Read the model definition and answer for the solid it produces. Units are mm, in the model's axes. A direction names the side the tool comes from. Coordinates: 2 decimals unless noted, no trailing zeros. Loops run counter-clockwise (first coordinate to the right, second up) from the corner with the lowest first, then second, coordinate; pieces in that order, holes last. Notation, with made-up numbers: (-4.75, 25.5) -> (15.25, 25.5) arc R3 ccw to (15.25, 30.5) -> close; hole circle Ø3 at (56, -34). An arc over 180 degrees is marked (long way). Answer in a Markdown table with one row per item.
```python
from build123d import *

# Parameters (mm, degrees)
SKETCH_1_R          = 10
SKETCH_1_R_2        = 1.65
EXTRUDE_1_DEPTH     = 3
SKETCH_2_R          = 3
EXTRUDE_2_DEPTH     = 80
CUT_EXTRUDE_1_DEPTH = 20


with BuildPart() as part:
    # 草图1 → 凸台-拉伸1 (new body)
    with BuildSketch(Plane.XY):
        Circle(SKETCH_1_R)
        with Locations((0, 7)):
            Circle(SKETCH_1_R_2, mode=Mode.SUBTRACT)
        with Locations((7, 0)):
            Circle(SKETCH_1_R_2, mode=Mode.SUBTRACT)
        with Locations((0, -7)):
            Circle(SKETCH_1_R_2, mode=Mode.SUBTRACT)
        with Locations((-7, 0)):
            Circle(SKETCH_1_R_2, mode=Mode.SUBTRACT)
    extrude(amount=EXTRUDE_1_DEPTH)

    # 草图2 → 凸台-拉伸2 (add)
    with BuildSketch(Plane.XY.offset(3)):
        Circle(SKETCH_2_R)
    extrude(amount=EXTRUDE_2_DEPTH)

    # 草图3 → 切除-拉伸1 (cut)
    with BuildSketch(Plane.XY.offset(83)):
        with BuildLine():
            Line((-0.75, 1.299038106), (-0.75, 2.25))
            Line((-0.75, 2.25), (0.75, 2.25))
            Line((0.75, 2.25), (0.75, 1.299038106))
            ThreePointArc((0.75, 1.299038106), (0, -1.5), (-0.75, 1.299038106))
        make_face()
    extrude(amount=-CUT_EXTRUDE_1_DEPTH, mode=Mode.SUBTRACT)


solid = part.part
```
1. Given pin 1 Ø4 at (y, z) = (5.5, 58.5) entering from +X; pin 2 Ø1 at (y, z) = (2, 76) entering from +X; pin 3 Ø5 at (y, z) = (0, 57) entering from -X; pin 4 Ø0.8 at (y, z) = (1.5, 72.5) entering from -X, each flat-ended and moving along its own axis, determine where each tip first touches the part or whether it passes through.
A:
| item | result |
|---|---|
| pin 1 | passes through |
| pin 2 | stops at x = 2.6 |
| pin 3 | stops at x = -3 |
| pin 4 | stops at x = -2.79 |
2. Find the intervals of material crossed by probe 1 along Y at (x, z) = (0, 68.75); probe 2 along Y at (x, z) = (0, 1.75); probe 3 along Z at (x, y) = (1.75, 4.5), in increasing order.
A:
| item | result |
|---|---|
| probe 1 | y = -3 to -1.5, 2.25 to 3 |
| probe 2 | y = -10 to -8.65, -5.35 to 5.35, 8.65 to 10 |
| probe 3 | z = 0 to 3 |
3. The mould has two halves that part along X. Classify faces 3 (the cylindrical face through (-3, 0, 42)), 4 (the cylindrical face through (-0.4, 5.4, 1.5)), 5 (the flat face through (0, 0, 0)): pulls with the +X half, pulls with the -X half, needs draft (parallel to the pull), parting line crosses it, or undercut.
A:
| item | result |
|---|---|
| face 3 | parting line crosses it |
| face 4 | undercut |
| face 5 | needs draft |
4. A cutting plane is placed at D-D on z = 51.5. Give the vertices of the cut face in (x, y).
A:
| item | result |
|---|---|
| outline | circle Ø6 at (0, 0) |
5. A cutting plane is placed at C-C on y = 6.25. Give the vertices of the cut face in (x, z).
A:
| item | result |
|---|---|
| outline | (-7.81, 0) -> (-1.47, 0) -> (-1.47, 3) -> (-7.81, 3) -> close; (1.47, 0) -> (7.81, 0) -> (7.81, 3) -> (1.47, 3) -> close |
6. A tool of negligible diameter and unlimited length cuts with its end or side. For faces 1 (the cylindrical face through (-8.65, 0.07, 1.48)), 2 (the flat face through (0, 2.25, 73)), from which of +Z, -Z, +X, -X, +Y, -Y can it reach the whole face along a straight path? Write none if from no direction.
A:
| item | result |
|---|---|
| face 1 | +Z, -Z |
| face 2 | +Z |
7. A cutting plane is placed at B-B on x = -7.25. Give the vertices of the cut face in (y, z), and give its area (3 significant figures).
A:
| item | result |
|---|---|
| outline | (-6.89, 0) -> (-1.63, 0) -> (-1.63, 3) -> (-6.89, 3) -> close; (1.63, 0) -> (6.89, 0) -> (6.89, 3) -> (1.63, 3) -> close |
| area | 31.5 mm2 |
8. A cutting plane is placed at A-A on y = 0. Give the vertices of the cut face in (x, z).
A:
| item | result |
|---|---|
| outline | (-10, 0) -> (-8.65, 0) -> (-8.65, 3) -> (-10, 3) -> close; (-5.35, 0) -> (5.35, 0) -> (5.35, 3) -> (3, 3) -> (3, 83) -> (1.5, 83) -> (1.5, 63) -> (-1.5, 63) -> (-1.5, 83) -> (-3, 83) -> (-3, 3) -> (-5.35, 3) -> close; (8.65, 0) -> (10, 0) -> (10, 3) -> (8.65, 3) -> close |
